The model under review builds one solid part; all positions refer to its coordinate system, in mm. A direction names the side the tool comes from. Give positions to 0.01 mm unless a question says otherwise; leave off trailing zeros. Write each loop counter-clockwise with the first axis right and the second up, starting at its lowest first coordinate (ties: lowest second). Pieces come first, ordered by that corner, then holes. Notation, with made-up numbers: (78, 86.25) -> (117, 86.25) arc R11 ccw to (117, 103.25) -> close; hole circle Ø10 at (30.25, -17). An arc over 180 degrees is marked (long way). Use CSV: the item, a comma, the result in double quotes.
```python
from build123d import *

# Parameters (mm, degrees)
SKETCH1_R           = 2.5
BOSS_EXTRUDE1_DEPTH = 16
CHAMFER1_SIZE       = 0.5
BOSS_EXTRUDE2_DEPTH = 3.5


with BuildPart() as part:
    # Sketch1 → Boss-Extrude1 (new body)
    with BuildSketch(Plane(origin=(0, 0, 0), x_dir=(1, 0, 0), z_dir=(0, 1, 0))):
        with Locations(Location((0, 0, 0), (0, 0, 270))):
            Circle(SKETCH1_R)
    extrude(amount=BOSS_EXTRUDE1_DEPTH)

    # Chamfer1
    chamfer1_edges = [part.edges().sort_by_distance(p)[0] for p in [
        (0, 16, -2.5),
    ]]
    chamfer(chamfer1_edges, length=CHAMFER1_SIZE)

    # Sketch2 → Boss-Extrude2 (add)
    with BuildSketch(Plane.XZ):
        Polygon((4.595076966, 0.467547866), (1.892630154, 4.213227318), (-2.702446812, 3.745679452), (-4.595076966, -0.467547866), (-1.892630154, -4.213227318), (2.702446812, -3.745679452), align=None)
    extrude(amount=BOSS_EXTRUDE2_DEPTH)

    # Sketch4 → Cut-Revolve1 (revolve, cut)
    with BuildSketch(Plane(origin=(0, 0, 0), x_dir=(0, 0, -1), z_dir=(1, 0, 0))):
        Polygon((0, -3.5), (2.5, -3.5), (6.193754438, -2.155583332), (6.193754438, -4.64679672), (0, -4.64679672), align=None)
    revolve(axis=Axis((0, 0, 0), (0, -1, 0)), mode=Mode.SUBTRACT)


solid = part.part
```
Q1. Consider section C-C (x = 0). Write out the cut boundary in (y, z).
Derived:
outline,"(-3.5, -2.5) -> (-2.95, -4.02) -> (0, -4.02) -> (0, -2.5) -> (15.5, -2.5) -> (16, -2) -> (16, 2) -> (15.5, 2.5) -> (0, 2.5) -> (0, 4.02) -> (-2.95, 4.02) -> (-3.5, 2.5) -> close"
Q2. To check wall thickness, follow probe 1 along X at (y, z) = (8.25, 1.5); probe 2 along X at (y, z) = (1, 0); probe 3 along Y at (x, z) = (2.25, 2). State the ranges of each line that lie inside material, in increasing order.
Derived:
probe 1,"x = -2 to 2"
probe 2,"x = -2.5 to 2.5"
probe 3,"y = -3.31 to 0"
Q3. Machinability: for faces 1 (the cylindrical face through (-2.44, 7.64, -0.54)), 2 (the flat face through (0, 16, 0)), which of the approach directions +Z, -Z, +X, -X, +Y, -Y give a long, thin tool a straight path to every point of the face, cutting with its end or side? Answer none if there is none.
Derived:
face 1,"+Y"
face 2,"+Z, -Z, +X, -X, +Y"
Q4. Consider section A-A (z = 0). Write out the cut boundary in (x, y), then the cut area to 3 significant figures.
Derived:
outline,"(-4.39, -2.81) -> (-2.5, -3.5) -> (2.5, -3.5) -> (4.39, -2.81) -> (4.39, 0) -> (2.5, 0) -> (2.5, 15.5) -> (2, 16) -> (-2, 16) -> (-2.5, 15.5) -> (-2.5, 0) -> (-4.39, 0) -> close"
area,"109 mm2"
Q5. Consider section B-B (y = 6). Write out the cut boundary in (x, z), then the cut area to 3 significant figures.
Derived:
outline,"circle Ø5 at (0, 0)"
area,"19.6 mm2"
